```python
from build123d import *

# Parameters (mm, degrees)
SKETCH1_W              = 190.5
SKETCH1_H              = 209.55
SKETCH1_W_2            = 165.1
SKETCH1_H_2            = 184.15
BOSS_EXTRUDE2_DEPTH    = 5.08
F_10_32_TAPPED_HOLE1_D = 4.0386
FILLET1_R              = 6.35


with BuildPart() as part:
    # Sketch1 → Boss-Extrude2 (new body)
    with BuildSketch(Plane(origin=(0, 0, 0), x_dir=(0, 0, -1), z_dir=(1, 0, 0))):
        with Locations((95.25, 104.775)):
            Rectangle(SKETCH1_W, SKETCH1_H)
        with Locations((95.25, 104.775)):
            Rectangle(SKETCH1_W_2, SKETCH1_H_2, mode=Mode.SUBTRACT)
    extrude(amount=BOSS_EXTRUDE2_DEPTH)

    # #10-32 Tapped Hole1 (through all)
    with Locations(Plane(origin=(5.08, 0, 0), x_dir=(0, 0, -1), z_dir=(1, 0, 0))):
        with Locations((6.35, 203.2), (184.15, 6.35), (6.35, 6.35), (184.15, 203.2), (95.25, 6.35), (95.25, 203.2), (6.35, 137.583333333), (6.35, 71.966666667), (184.15, 71.966666667), (184.15, 137.583333333)):
            Hole(F_10_32_TAPPED_HOLE1_D / 2)

    # Fillet1
    fillet1_edges = [part.edges().sort_by_distance(p)[0] for p in [
        (2.54, 196.85, -12.7),
        (2.54, 12.7, -12.7),
        (2.54, 12.7, -177.8),
        (2.54, 196.85, -177.8),
        (2.54, 209.55, 0),
        (2.54, 209.55, -190.5),
        (2.54, 0, -190.5),
        (2.54, 0, 0),
    ]]
    fillet(fillet1_edges, radius=FILLET1_R)


solid = part.part
```
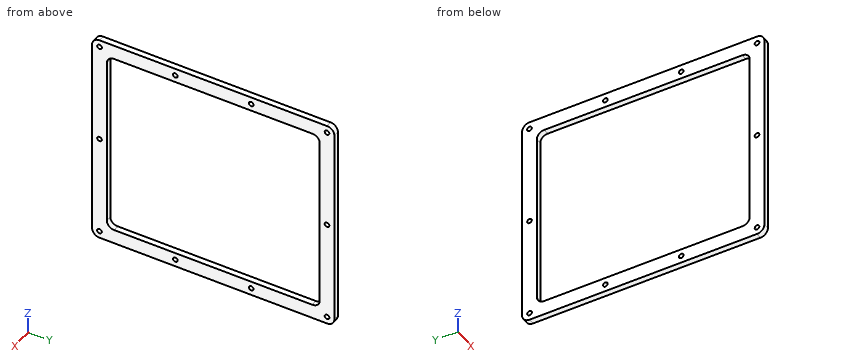
Work out the finished part from the listing and answer in its coordinate system (mm). Give positions to 0.01 mm unless a question says otherwise; leave off trailing zeros. Loops run counter-clockwise (first coordinate to the right, second up) from the corner with the lowest first, then second, coordinate; pieces in that order, holes last. Notation, with made-up numbers: (-36, -6.75) -> (-28, -6.75) arc R20 cw to (-28, -2.75) -> close; hole circle Ø3 at (-22, 80.5). An arc over 180 degrees is marked (long way). Use CSV: the item, a comma, the result in double quotes.
1. Straight lines are drawn through the part: line 1 (Y direction, x = 2.8, z = -95.25); line 2 (Z direction, x = 3.15, y = 26.5); line 3 (Y direction, x = 2.05, z = -63.5). For each, find the intervals that lie inside material, in ascending order.
Found:
line 1,"0 to 4.33, 8.37 to 12.7, 196.85 to 201.18, 205.22 to 209.55"
line 2,"-190.5 to -177.8, -12.7 to 0"
line 3,"0 to 12.7, 196.85 to 209.55"
2. The part is cut by section B-B (y = 142). Write down the section's boundary in (x, z).
Found:
outline,"(0, -190.5) -> (5.08, -190.5) -> (5.08, -177.8) -> (0, -177.8) -> close; (0, -12.7) -> (5.08, -12.7) -> (5.08, 0) -> (0, 0) -> close"
3. The part is cut by section A-A (z = -61). Write down the section's boundary in (x, y), then the cut area to 3 significant figures.
Found:
outline,"(0, 0) -> (5.08, 0) -> (5.08, 12.7) -> (0, 12.7) -> close; (0, 196.85) -> (5.08, 196.85) -> (5.08, 209.55) -> (0, 209.55) -> close"
area,"129 mm^2"
4. The part is cut by section C-C (x = 2.95). State how many separate pieces and enclosed holes the cut face has, then the cut area to 3 significant figures.
Found:
separate pieces,"1"
enclosed holes,"11"
area,"9,390 mm^2"
